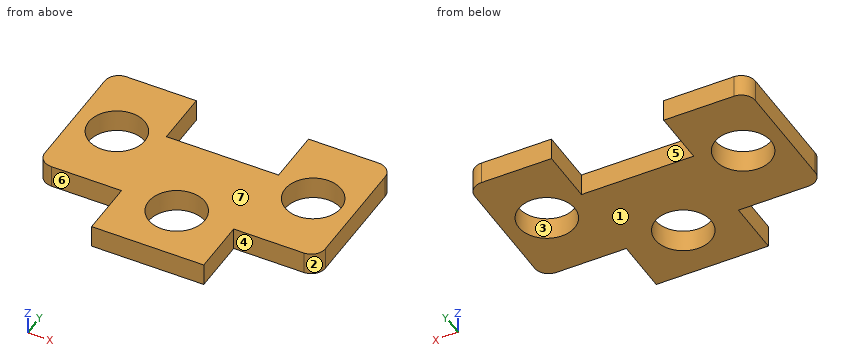
from build123d import *

# Parameters (mm, degrees)
SKETCH1_R           = 50
BOSS_EXTRUDE1_DEPTH = 40


with BuildPart() as part:
    # Sketch1 → Boss-Extrude1 (new body)
    with BuildSketch(Plane.XY):
        with BuildLine():
            Line((-100, -122.09449171), (-100, -222.09449171))
            Line((-100, -222.09449171), (100, -222.09449171))
            Line((100, -222.09449171), (100, -122.09449171))
            Line((100, -122.09449171), (225, -122.09449171))
            ThreePointArc((225, -122.09449171), (242.67766953, -114.772161239), (250, -97.09449171))
            Line((250, -97.09449171), (250, 102.90550829))
            ThreePointArc((250, 102.90550829), (242.67766953, 120.58317782), (225, 127.90550829))
            Line((225, 127.90550829), (100, 127.90550829))
            Line((100, 127.90550829), (100, 27.90550829))
            Line((100, 27.90550829), (-100, 27.90550829))
            Line((-100, 27.90550829), (-100, 127.90550829))
            Line((-100, 127.90550829), (-225, 127.90550829))
            ThreePointArc((-225, 127.90550829), (-242.67766953, 120.58317782), (-250, 102.90550829))
            Line((-250, 102.90550829), (-250, -97.09449171))
            ThreePointArc((-250, -97.09449171), (-242.67766953, -114.772161239), (-225, -122.09449171))
            Line((-225, -122.09449171), (-100, -122.09449171))
        make_face()
        with Locations((0, -125)):
            Circle(SKETCH1_R, mode=Mode.SUBTRACT)
        with Locations((175, 2.90550829)):
            Circle(SKETCH1_R, mode=Mode.SUBTRACT)
        with Locations(Location((-175, 2.90550829, 0), (0, 0, 180))):
            Circle(SKETCH1_R, mode=Mode.SUBTRACT)
    extrude(amount=BOSS_EXTRUDE1_DEPTH)


solid = part.part
Source: CAD feature listing. Evaluate the final solid. Frame: model axes, mm. Face numbers are marked on the shaded views. A direction names the side the tool comes from. Give positions to 0.01 mm unless a question says otherwise; leave off trailing zeros. Loops run counter-clockwise (first coordinate to the right, second up) from the corner with the lowest first, then second, coordinate; pieces in that order, holes last. Notation, with made-up numbers: (10, -0.5) -> (43, -0.5) arc R20 ccw to (43, 30.5) -> close; hole circle Ø5 at (44, 21). An arc over 180 degrees is marked (long way). Use a Markdown table: item, result. Add a question column.
1) Line query: line 1 along X through (y, z) = (2, 5.5); line 2 along X through (y, z) = (91.5, 2); line 3 along Y through (x, z) = (-3, 15). Output: solid intervals per line, ascending. Write a range as [from, to].
2) Section query C-C, the plane y = -22.5. Return the cut outline in (x, z).
3) Pull-direction query (Y, two-part tool) for the marked faces 1, 2 and 3; classes: +Y half, -Y half, draft (parallel to the pull), parting line (faces both ways), or undercut.
4) Reachability of the marked faces 4, 5, 6 and 7 from +Z, -Z, +X, -X, +Y, -Y: full face, straight path, thin tool, end or side. Return the list, or none.
5) Section query D-D, the plane z = 30.5. Return the cut outline in (x, y), then the cut area to 3 significant figures.
6) Section query A-A, the plane x = 175. Return the cut outline in (y, z).
7) Section query B-B, the plane y = -133. Return the cut outline in (x, z), then the cut area to 3 significant figures.
8) First-contact query: pin 1 (3 mm diameter, centred on y = -168, z = 34, fed in from +X); pin 2 (8 mm diameter, centred on x = 74.5, z = 21, fed in from +Y); pin 3 (10 mm diameter, centred on y = -151, z = 16, fed in from -X); pin 4 (4 mm diameter, centred on x = 64.5, y = -94, fed in from -Z). Flat tips, straight axial feed; report the tip coordinate or a pass-through.
Numbers:
| question | item | result |
|---|---|---|
| 1 | line 1 | x = [-250, -224.99], [-125.01, 125.01], [224.99, 250] |
| 1 | line 2 | x = [-250, -100], [100, 250] |
| 1 | line 3 | y = [-222.09, -174.91], [-75.09, 27.91] |
| 2 | outline | (-250, 0) -> (-218.06, 0) -> (-218.06, 40) -> (-250, 40) -> close; (-131.94, 0) -> (131.94, 0) -> (131.94, 40) -> (-131.94, 40) -> close; (218.06, 0) -> (250, 0) -> (250, 40) -> (218.06, 40) -> close |
| 3 | face 1 | draft |
| 3 | face 2 | -Y half |
| 3 | face 3 | undercut |
| 4 | face 4 | +Z, -Z, +X, -Y |
| 4 | face 5 | +Z, -Z, +Y |
| 4 | face 6 | +Z, -Z, -X, -Y |
| 4 | face 7 | +Z, +X, -X, +Y, -Y |
| 5 | outline | (-250, -97.09) arc R25 ccw to (-225, -122.09) -> (-100, -122.09) -> (-100, -222.09) -> (100, -222.09) -> (100, -122.09) -> (225, -122.09) arc R25 ccw to (250, -97.09) -> (250, 102.91) arc R25 ccw to (225, 127.91) -> (100, 127.91) -> (100, 27.91) -> (-100, 27.91) -> (-100, 127.91) -> (-225, 127.91) arc R25 ccw to (-250, 102.91) -> close; hole circle Ø100 at (-175, 2.91); hole circle Ø100 at (0, -125); hole circle Ø100 at (175, 2.91) |
| 5 | area | 101,000 mm2 |
| 6 | outline | (-122.09, 0) -> (-47.09, 0) -> (-47.09, 40) -> (-122.09, 40) -> close; (52.91, 0) -> (127.91, 0) -> (127.91, 40) -> (52.91, 40) -> close |
| 7 | outline | (-100, 0) -> (-49.36, 0) -> (-49.36, 40) -> (-100, 40) -> close; (49.36, 0) -> (100, 0) -> (100, 40) -> (49.36, 40) -> close |
| 7 | area | 4,050 mm2 |
| 8 | pin 1 | stops at x = 100 |
| 8 | pin 2 | stops at y = 27.91 |
| 8 | pin 3 | stops at x = -100 |
| 8 | pin 4 | stops at z = 0 |
